CAD build for the part. Positions are in the model's coordinates, mm. A direction names the side the tool comes from. Round coordinates to 2 decimals unless told otherwise and drop trailing zeros. Order: outer loops, then holes, each group sorted by start corner. A loop starts at its lowest first (then second) coordinate and runs counter-clockwise, first axis right, second up. Notation, with made-up numbers: M 89,29 L 109,29 A35 ccw 109,64 Z; hole C 8,51.5 d4. An arc over 180 degrees is marked long. Answer as a JSON object with one key per item and string values.
```python
from build123d import *

# Parameters (mm, degrees)
BOSS_EXTRUDE1_DEPTH = 10
CHAMFER1_SIZE       = 1


with BuildPart() as part:
    # Sketch1 → Boss-Extrude1 (new body)
    with BuildSketch(Plane.XY):
        with BuildLine():
            ThreePointArc((4.371766903777949, 61.5450849718747), (3.661569294176898, 57.06107373853762), (-0.38351567769782763, 55))
            Line((-0.38351567769782763, 55), (-19.078784028338333, 54.99999999999999))
            Line((-19.078784028338333, 55.0000000000002), (-68.51590932319446, 30.505248230686387))
            ThreePointArc((-68.51590932319446, 30.50524823068639), (-72.64180115025157, 15.440491486016093), (-75.00000000000001, 7.8515e-13))
            Line((-75.00000000000001, 7.8558e-13), (-61.545084971874644, 4.371766903778592))
            ThreePointArc((-61.545084971874644, 4.37176690377859), (-57.06107373853757, 3.6615692941774913), (-55, -0.38351567769725153))
            Line((-55.00000000000001, -0.38351567769725153), (-55.000000000000135, -19.078784028338532))
            Line((-55.000000000000135, -19.078784028338532), (-30.50524823068615, -68.51590932319456))
            ThreePointArc((-30.505248230686153, -68.51590932319459), (-15.440491486015834, -72.64180115025164), (-5.2403e-13, -75.00000000000003))
            Line((-5.2372e-13, -75.00000000000001), (-4.371766903778377, -61.54508497187467))
            ThreePointArc((-4.371766903778381, -61.54508497187467), (-3.661569294177295, -57.061073738537594), (0.38351567769744355, -55))
            Line((0.38351567769744355, -55.00000000000001), (19.078784028338724, -55.00000000000007))
            Line((19.078784028338724, -55.00000000000007), (68.51590932319466, -30.50524823068591))
            ThreePointArc((68.51590932319468, -30.505248230685908), (72.64180115025168, -15.440491486015581), (75.00000000000001, -2.6112e-13))
            Line((75.00000000000001, -2.6186e-13), (61.54508497187469, -4.371766903778163))
            ThreePointArc((61.54508497187469, -4.371766903778164), (57.06107373853761, -3.6615692941770925), (55, 0.3835156776976356))
            Line((55.00000000000001, 0.3835156776976356), (55, 19.078784028338916))
            Line((55, 19.078784028338916), (30.50524823068567, 68.51590932319478))
            ThreePointArc((30.50524823068567, 68.51590932319476), (15.440491486015329, 72.64180115025172), (0, 75))
            Line((0, 75.00000000000001), (4.371766903777948, 61.5450849718747))
        make_face()
        with BuildLine():
            Line((16.12078785321155, -16.235544436876165), (13.522711641858239, -14.735544436876154))
            ThreePointArc((13.52271164185824, -14.735544436876154), (-6.000000000000136, -19.078784028338873), (-19.522711641858354, -4.343239591462642))
            ThreePointArc((-19.52271164185835, -4.343239591462641), (-13.522711641858244, 14.735544436876156), (6.000000000000001, 19.078784028338916))
            ThreePointArc((5.999999999999998, 19.078784028338916), (17.320508075688796, 9.999999999999961), (19.522711641858287, -4.3432395914629165))
            Line((19.522711641858287, -4.343239591462916), (22.1207878532116, -5.843239591462927))
            Line((22.1207878532116, -5.843239591462927), (16.12078785321155, -16.235544436876165))
        make_face(mode=Mode.SUBTRACT)
    extrude(amount=-BOSS_EXTRUDE1_DEPTH)

    # Chamfer1
    chamfer1_edges = [part.edges().sort_by_distance(p)[0] for p in [
        (-19.522711641858322, -4.343239591462766, 0),
        (-19.522711641858322, -4.343239591462773, -10),
    ]]
    chamfer(chamfer1_edges, length=CHAMFER1_SIZE)


solid = part.part
```
Item 1: Saw through at B-B on y = 34.5. List the corners of the cut face in (x, z), and give its area (3 significant figures).
Worked answers:
{"outline": "M -60.45,-10 L 47.36,-10 L 47.36,0 L -60.45,0 Z", "area": "1,080 mm2"}
Item 2: Saw through at C-C on y = -35. List the corners of the cut face in (x, z).
Worked answers:
{"outline": "M -47.11,-10 L 59.44,-10 L 59.44,0 L -47.11,0 Z"}
Item 3: Two-plate mould, pull along X, no slides. Class faces 1 (the flat face through (-18, 18, 0)), 2 (the cylindrical face through (15.654, 72.596, -4.93)), 3 (the flat face through (68.367, -2.155, -4.93)): released by +X, released by -X, zero draft, split by the parting line, or undercut.
Worked answers:
{"face 1": "zero draft", "face 2": "released by +X", "face 3": "undercut"}
Item 4: 3-axis set-ups, long thin cutter, end or side, ignore diameter. For faces 4 (the flat face through (2.155, 68.367, -4.93)), 5 (the conical face through (-17.86, 9.381, -9.174)), 6 (the flat face through (10, -55, -5)), 7 (the flat face through (19.16, -10.97, -4.93)), 8 (the flat face through (-10, 55, -5)): which of +Z, -Z, +X, -X, +Y, -Y reach the whole face in a straight line?
Worked answers:
{"face 4": "+Z, -Z, -X", "face 5": "-Z", "face 6": "+Z, -Z, +X, -Y", "face 7": "+Z, -Z", "face 8": "+Z, -Z, -X, +Y"}
Item 5: Saw through at A-A on z = -2.75. List the corners of the cut face in (x, y).
Worked answers:
{"outline": "M -75,0 L -61.55,4.37 A5 cw -55,-0.38 L -55,-19.08 L -30.51,-68.52 A135 ccw 0,-75 L -4.37,-61.55 A5 cw 0.38,-55 L 19.08,-55 L 68.52,-30.51 A135 ccw 75,0 L 61.55,-4.37 A5 cw 55,0.38 L 55,19.08 L 30.51,68.52 A135 ccw 0,75 L 4.37,61.55 A5 cw -0.38,55 L -19.08,55 L -68.52,30.51 A135 ccw Z; hole M 13.52,-14.74 L 16.12,-16.24 L 22.12,-5.84 L 19.52,-4.34 A20 ccw long Z"}
Item 6: Wall check: line 1 along Y through (x, z) = (-12, -9); line 2 along X through (y, z) = (-67.5, -3.75); line 3 along X through (y, z) = (-43.5, -7.5). Give the ranges that are in metal, low to high. Write a range as [from, to].
Worked answers:
{"line 1": "y = [-73.33, -16], [16, 55]", "line 2": "x = [-31.01, -2.44]", "line 3": "x = [-42.9, 42.29]"}
Item 7: Drop flat-ended pins along their axis: pin 1 Ø4 at (y, z) = (-44.5, -2.5) entering from -X; pin 2 Ø4 at (x, z) = (7, -8.5) entering from +Y; pin 3 Ø5 at (y, z) = (13, -3.5) entering from +X. Give the stop position or say it passes through.
Worked answers:
{"pin 1": "stops at x = -43.4", "pin 2": "stops at y = 74.44", "pin 3": "stops at x = 55"}
